```python
from build123d import *

# Parameters (mm, degrees)
SKETCH1_W           = 70
SKETCH1_H           = 70
SKETCH1_R           = 2.6
BOSS_EXTRUDE1_DEPTH = 12.5
SKETCH2_R           = 27.5
CUT_EXTRUDE1_DEPTH  = 14
FILLET1_R           = 0.8
BOSS_EXTRUDE2_DEPTH = 1.5
SKETCH5_W           = 30
SKETCH5_H           = 8
CUT_EXTRUDE2_DEPTH  = 80.504716841
SKETCH6_W           = 30
SKETCH6_H           = 8
CUT_EXTRUDE3_DEPTH  = 80.504716841


with BuildPart() as part:
    # Sketch1 → Boss-Extrude1 (new body)
    with BuildSketch(Plane(origin=(0, 0, 0), x_dir=(1, 0, 0), z_dir=(0, 1, 0))):
        Rectangle(SKETCH1_W, SKETCH1_H)
        with Locations(Location((31.5, 31.5, 0), (0, 0, 270))):
            Circle(SKETCH1_R, mode=Mode.SUBTRACT)
        with Locations(Location((-31.5, 31.5, 0), (0, 0, 270))):
            Circle(SKETCH1_R, mode=Mode.SUBTRACT)
        with Locations(Location((31.5, -31.5, 0), (0, 0, 270))):
            Circle(SKETCH1_R, mode=Mode.SUBTRACT)
        with Locations(Location((-31.5, -31.5, 0), (0, 0, 270))):
            Circle(SKETCH1_R, mode=Mode.SUBTRACT)
    extrude(amount=BOSS_EXTRUDE1_DEPTH)

    # Sketch2 → Cut-Extrude1 (cut)
    with BuildSketch(Plane(origin=(0, 12.5, 0), x_dir=(1, 0, 0), z_dir=(0, 1, 0))):
        with Locations(Location((0, 0, 0), (0, 0, 270))):
            Circle(SKETCH2_R)
    extrude(amount=-CUT_EXTRUDE1_DEPTH, mode=Mode.SUBTRACT)

    # Fillet1
    fillet1_edges = [part.edges().sort_by_distance(p)[0] for p in [
        (0, 12.5, -27.5),
    ]]
    fillet(fillet1_edges, radius=FILLET1_R)

    # Sketch3 → Boss-Extrude2 (add)
    with BuildSketch(Plane(origin=(0, 12.5, 0), x_dir=(1, 0, 0), z_dir=(0, 1, 0))):
        Polygon((33.6, 17.9), (21.6, 17.9), (20.8, 18.7), (34.4, 18.7), align=None)
        Polygon((33.6, -17.9), (21.6, -17.9), (20.8, -18.7), (34.4, -18.7), align=None)
    extrude(amount=BOSS_EXTRUDE2_DEPTH)

    # Sketch5 → Cut-Extrude2 (cut, through all)
    with BuildSketch(Plane.XY.offset(35)):
        with Locations((0, 6.25)):
            Rectangle(SKETCH5_W, SKETCH5_H)
    extrude(amount=-CUT_EXTRUDE2_DEPTH, mode=Mode.SUBTRACT)

    # Sketch6 → Cut-Extrude3 (cut, through all)
    with BuildSketch(Plane(origin=(35, 0, 0), x_dir=(0, 0, -1), z_dir=(1, 0, 0))):
        with Locations((0, 6.25)):
            Rectangle(SKETCH6_W, SKETCH6_H)
    extrude(amount=-CUT_EXTRUDE3_DEPTH, mode=Mode.SUBTRACT)


solid = part.part
```
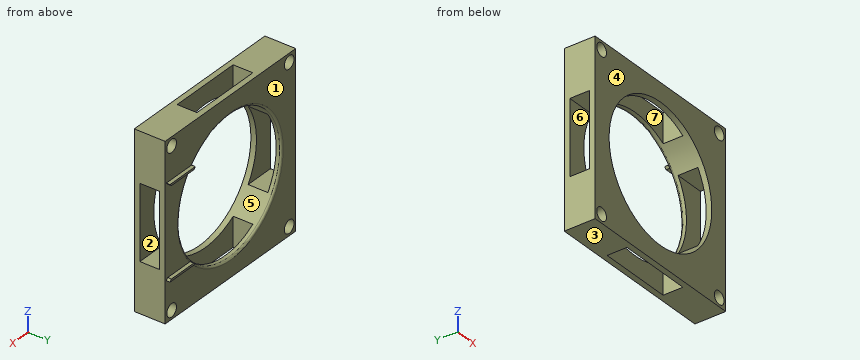
Geometry check sheet. Reference: the model listing, model coordinates, mm. Face numbers are marked on the shaded views. A direction names the side the tool comes from. Round coordinates to 2 decimals unless told otherwise and drop trailing zeros. Loops run counter-clockwise (first coordinate to the right, second up) from the corner with the lowest first, then second, coordinate; pieces in that order, holes last. Notation, with made-up numbers: (-34, -17.5) - (-15, -17.5) arc R36 cw to (-15, 20.5) - close; hole circle Ø7 at (11.5, -26). An arc over 180 degrees is marked (long way). Write item = value, one per line. Start each with the question number.
1. Section check C-C on x = 31.5. Enter the section's corners in (y, z), then the cut area to 3 significant figures.
2. Section check D-D on z = 8. Give the number of separate pieces and of enclosed holes in the cut face, then the cut area to 3 significant figures.
3. Section check B-B on x = -31.5. Enter the section's corners in (y, z).
4. Section check A-A on y = 8.5. Enter the section's corners in (x, z).
5. Depth check by flat-ended pin: pin 1 (0.8 mm diameter, centred on x = 26.5, y = 13.5, fed in from -Z); pin 2 (12 mm diameter, centred on x = -8.5, z = -20, fed in from +Y); pin 3 (9.5 mm diameter, centred on x = -3, z = -29.5, fed in from +Y); pin 4 (4 mm diameter, centred on x = -31.5, z = -31.5, fed in from +Y). Enter the tip coordinate at first touch or a pass-through.
6. Mould release check, pull along Z, two halves, no side actions. Record for the marked faces 1, 2, 3 and 4: released by +Z, released by -Z, zero draft, split by the parting line, or undercut.
7. Set-up check for the marked faces 5, 6 and 7: record each of +Z, -Z, +X, -X, +Y, -Y from which the full face is reachable in a straight line by a thin tool's end or side.
8. Thickness scan on line 1 (X direction, y = 7.5, z = -31.5); line 2 (Y direction, x = 10, z = -31.5); line 3 (Z direction, x = -23.5, y = 7.5). Record the ranges inside material, lowest first.
Working result:
q1.outline = (0, -35) - (12.5, -35) - (12.5, -34.1) - (0, -34.1) - close; (0, -28.9) - (12.5, -28.9) - (12.5, -18.7) - (14, -18.7) - (14, -17.9) - (12.5, -17.9) - (12.5, 17.9) - (14, 17.9) - (14, 18.7) - (12.5, 18.7) - (12.5, 28.9) - (0, 28.9) - close; (0, 34.1) - (12.5, 34.1) - (12.5, 35) - (0, 35) - close; hole (2.25, -15) - (10.25, -15) - (10.25, 15) - (2.25, 15) - close
q1.area = 507 mm^2
q2.separate_pieces = 4
q2.enclosed_holes = 0
q2.area = 77.9 mm^2
q3.outline = (0, -35) - (12.5, -35) - (12.5, -34.1) - (0, -34.1) - close; (0, -28.9) - (12.5, -28.9) - (12.5, 28.9) - (0, 28.9) - close; (0, 34.1) - (12.5, 34.1) - (12.5, 35) - (0, 35) - close; hole (2.25, -15) - (10.25, -15) - (10.25, 15) - (2.25, 15) - close
q4.outline = (-35, -35) - (-15, -35) - (-15, -23.05) arc R27.5 cw to (-23.05, -15) - (-35, -15) - close; (-35, 15) - (-23.05, 15) arc R27.5 cw to (-15, 23.05) - (-15, 35) - (-35, 35) - close; (15, -35) - (35, -35) - (35, -15) - (23.05, -15) arc R27.5 cw to (15, -23.05) - close; (15, 23.05) arc R27.5 cw to (23.05, 15) - (35, 15) - (35, 35) - (15, 35) - close; hole circle Ø5.2 at (-31.5, -31.5); hole circle Ø5.2 at (-31.5, 31.5); hole circle Ø5.2 at (31.5, -31.5); hole circle Ø5.2 at (31.5, 31.5)
q5.pin_1 = -18.7
q5.pin_2 = 12.26
q5.pin_3 = 12.5
q5.pin_4 = through
q6.face_1 = undercut
q6.face_2 = undercut
q6.face_3 = released by -Z
q6.face_4 = zero draft
q7.face_5 = +Y, -Y
q7.face_6 = +X, -X
q7.face_7 = +Z, -Z
q8.line_1 = -35 to -34.1, -28.9 to -15, 15 to 28.9, 34.1 to 35
q8.line_2 = 0 to 2.25, 10.25 to 12.5
q8.line_3 = -35 to -15, 15 to 35
